Verification items for the finished model (mm, model axes). A direction names the side the tool comes from. Round coordinates to 2 decimals unless told otherwise and drop trailing zeros. Write each loop counter-clockwise with the first axis right and the second up, starting at its lowest first coordinate (ties: lowest second). Pieces come first, ordered by that corner, then holes. Notation, with made-up numbers: (-31.5, -25.75) - (4.5, -25.75) arc R11 ccw to (4.5, -19.75) - close; hole circle Ø8 at (89.25, 21.25). An arc over 180 degrees is marked (long way). Answer as a JSON object with one key per item and string values. Group by question number.
1) Section check B-B (y = 15.5). Enter the section's corners in (x, z), then the cut area to 3 significant figures.
2) Mould release check, pull along X, two halves, no side actions. Record for faces 1 (the cylindrical face through (-25.773, 2.465, -11.358)), 2 (the cylindrical face through (-20.65, 8.38, -53.17)), 3 (the flat face through (-27, 0, -35)): +X half, -X half, draft (parallel to the pull), parting line (faces both ways), or undercut.
3) Thickness scan on line 1 (X direction, y = 3.9, z = -47.4); line 2 (X direction, y = 5.5, z = -47.5); line 3 (Y direction, x = -27.5, z = -10.5). Record the ranges inside material, lowest first.
4) Set-up check for faces 4 (the flat face through (-29, 5, -47)), 5 (the flat face through (-33.5, 8, -34)): record each of +Z, -Z, +X, -X, +Y, -Y from which the full face is reachable in a straight line by a thin tool's end or side.
5) Section check A-A (y = 1). Enter the section's corners in (x, z).
6) Section check D-D (z = -57). Enter the section's corners in (x, y).
7) Section check C-C (x = -28.5). Enter the section's corners in (y, z).
```python
from build123d import *

# Parameters (mm, degrees)
SKETCH_1_W          = 13.5
SKETCH_1_H          = 68.4
EXTRUDE_1_DEPTH     = 17
SKETCH_2_R          = 2.75
CUT_EXTRUDE_1_DEPTH = 5
CUT_EXTRUDE_2_DEPTH = 17
EXTRUDE_2_DEPTH     = 5.5
SKETCH_11_W         = 4
SKETCH_11_H         = 20
CUT_EXTRUDE_7_DEPTH = 17
FILLET_1_R          = 30
FILLET_2_R          = 1
SKETCH_7_W          = 30
SKETCH_7_H          = 69.053295448
CUT_EXTRUDE_4_DEPTH = 17


with BuildPart() as part:
    # ｽｹｯﾁ1 → ﾎﾞｽ - 押し出し1 (new body)
    with BuildSketch(Plane(origin=(0, 0, 0), x_dir=(1, 0, 0), z_dir=(0, 1, 0))):
        with Locations((6.75, 34.2)):
            Rectangle(SKETCH_1_W, SKETCH_1_H)
    extrude(amount=EXTRUDE_1_DEPTH)

    # ｽｹｯﾁ2 → ｶｯﾄ - 押し出し1 (cut)
    with BuildSketch(Plane.XZ):
        with Locations(Location((8.5, -47.4, 0), (0, 0, 270))):
            Circle(SKETCH_2_R)
        with Locations(Location((8.5, -11, 0), (0, 0, 90))):
            Circle(SKETCH_2_R)
    extrude(amount=-CUT_EXTRUDE_1_DEPTH, mode=Mode.SUBTRACT)

    # ｽｹｯﾁ3 → ｶｯﾄ - 押し出し2 (cut)
    with BuildSketch(Plane(origin=(0, 17, 0), x_dir=(1, 0, 0), z_dir=(0, 1, 0))):
        Polygon((6.75, 68.4), (0, 68.4), (0, 53.4), align=None)
    extrude(amount=-CUT_EXTRUDE_2_DEPTH, mode=Mode.SUBTRACT)

    # ｽｹｯﾁ4 → ﾎﾞｽ - 押し出し2 (add)
    with BuildSketch(Plane.XZ):
        Polygon((0, -47), (-4, -37), (-4, -27), (0, -27), align=None)
    extrude(amount=-EXTRUDE_2_DEPTH)

    # ｽｹｯﾁ11 → ｶｯﾄ - 押し出し7 (cut)
    with BuildSketch(Plane(origin=(0, 17, 0), x_dir=(1, 0, 0), z_dir=(0, 1, 0))):
        with Locations((-2, 37)):
            Rectangle(SKETCH_11_W, SKETCH_11_H)
    extrude(amount=-CUT_EXTRUDE_7_DEPTH, mode=Mode.SUBTRACT)

    # ﾌｨﾚｯﾄ1
    fillet_1_edges = [part.edges().sort_by_distance(p)[0] for p in [
        (0, 8.5, -53.4),
    ]]
    fillet(fillet_1_edges, radius=FILLET_1_R)

    # ﾌｨﾚｯﾄ2
    fillet_2_edges = [part.edges().sort_by_distance(p)[0] for p in [
        (6.75, 8.5, -68.4),
        (13.5, 8.5, -68.4),
        (13.5, 8.5, 0),
        (0, 8.5, 0),
    ]]
    fillet(fillet_2_edges, radius=FILLET_2_R)


with BuildPart() as body_2:
    # ﾐﾗｰ1: mirrored copy
    add(part.part.mirror(Plane.ZY.offset(10)))


with BuildPart() as part_1:
    add(part.part)

    # ｽｹｯﾁ7 → ｶｯﾄ - 押し出し4 (cut)
    with BuildSketch(Plane(origin=(0, 17, 0), x_dir=(1, 0, 0), z_dir=(0, 1, 0))):
        with Locations((-1.5, 34.526647724)):
            Rectangle(SKETCH_7_W, SKETCH_7_H)
    extrude(amount=-CUT_EXTRUDE_4_DEPTH, mode=Mode.SUBTRACT)


solid = body_2.part
```
Returned:
{
 "1": {"outline": "(-33.5, -67.4) arc R1 ccw to (-32.5, -68.4) - (-27.4, -68.4) arc R1 ccw to (-26.48, -67.81) - (-22.64, -59.27) arc R30 ccw to (-20, -46.96) - (-20, -1) arc R1 ccw to (-21, 0) - (-32.5, 0) arc R1 ccw to (-33.5, -1) - close", "area": "869 mm2"},
 "2": {"face 1": "undercut", "face 2": "+X half", "face 3": "draft"},
 "3": {"line 1": "-33.5 to -31.25, -25.75 to -20", "line 2": "-33.5 to -20", "line 3": "5 to 17"},
 "4": {"face 4": "-Y", "face 5": "+Z, -Z, -X, +Y, -Y"},
 "5": {"outline": "(-33.5, -67.4) arc R1 ccw to (-32.5, -68.4) - (-27.4, -68.4) arc R1 ccw to (-26.48, -67.81) - (-22.64, -59.27) arc R30 ccw to (-20, -46.96) - (-20, -1) arc R1 ccw to (-21, 0) - (-32.5, 0) arc R1 ccw to (-33.5, -1) - close; hole circle Ø5.5 at (-28.5, -47.4); hole circle Ø5.5 at (-28.5, -11)"},
 "6": {"outline": "(-33.5, 0) - (-21.73, 0) - (-21.73, 17) - (-33.5, 17) - close"},
 "7": {"outline": "(0, -68.4) - (17, -68.4) - (17, 0) - (0, 0) - (0, -8.25) - (5, -8.25) - (5, -13.75) - (0, -13.75) - (0, -44.65) - (5, -44.65) - (5, -50.15) - (0, -50.15) - close"}
}
